The listing builds one solid part. Answer for the finished solid, in the listing's coordinates (mm). Give positions to 0.01 mm unless a question says otherwise; leave off trailing zeros. Order: outer loops, then holes, each group sorted by start corner. A loop starts at its lowest first (then second) coordinate and runs counter-clockwise, first axis right, second up. Notation, with made-up numbers: (28.5, -22) - (47.5, -22) arc R35 cw to (47.5, 12) - close; hole circle Ø10 at (31, 6). An arc over 180 degrees is marked (long way). Answer as a JSON object with one key per item and string values. Group by question number.
Q1. Consider line 1 (Z direction, x = 0, y = -1.25); line 2 (Z direction, x = -0.5, y = 0.75); line 3 (Y direction, x = -0.25, z = -29). Determine where each line is inside the solid, lowest interval first.
Q2. A cutting plane is placed at C-C, the plane z = -16. Give the vertices of the cut face in (x, y).
Q3. A cutting plane is placed at B-B, the plane y = -1.75. Give the vertices of the cut face in (x, z) (3 decimals), and give its area (3 significant figures).
Q4. Given pin 1 (2 mm diameter, centred on y = 1, z = 25.5, fed in from +X), flat-ended and moving along its own axis, determine where the tip first touches the part or whether it passes through.
Q5. A cutting plane is placed at A-A, the plane x = 0. Give the vertices of the cut face in (y, z), and give its area (3 significant figures).
Q6. The mould has two halves that part along X. Classify faces 1 (the face through (-3.946, 0.174, 0.64)), 2 (the face through (0.172, 0.055, 43.855)), 3 (the face through (0, 0, -45.72)): released by +X, released by -X, zero draft, split by the parting line, or undercut.
Autodesk Inventor part; units mm, degrees
ref_plane "YZ Plane" through (0, 0, 0) normal (1, 0, 0) x (0, 1, 0)
ref_plane "XZ Plane" through (0, 0, 0) normal (0, 1, 0) x (-1, 0, 0)
ref_plane "XY Plane" through (0, 0, 0) normal (0, 0, 1) x (1, 0, 0)
sketch "Sketch1" plane through (0, 0, 0) normal (0, 0, 1) x (1, 0, 0)
  circle A0 centre (0, 0) radius 3.9497
  dimension "d0" = 7.8994
extrude "Extrusion1" add sketch "Sketch1" against normal mid plane 91.44
sketch "Sketch2" plane through (0, 0, 0) normal (0, 1, 0) x (-1, 0, 0)
  circle A0 centre (0, 42.545) radius 1.3208
  line L0 (-3.9497, 45.72) -> (3.9497, 45.72)
  point P0 (0, 45.72)
  dimension "d3" = 2.6416
  dimension "d4" = 3.175
extrude "Extrusion2" cut sketch "Sketch2" along normal through all both and the other way through all
mirror "Mirror1" about plane through (0, 0, 0) normal (0, 0, 1) of "Extrusion2"
properties part number "Handle_Rod" material "Steel, Mild"
Reply:
{
 "1": {"line 1": "z = -45.72 to -43.87, -41.22 to 41.22, 43.87 to 45.72", "line 2": "z = -45.72 to -43.77, -41.32 to 41.32, 43.77 to 45.72", "line 3": "y = -3.94 to 3.94"},
 "2": {"outline": "circle Ø7.9 at (0, 0)"},
 "3": {"outline": "(-3.541, -45.72) - (3.541, -45.72) - (3.541, 45.72) - (-3.541, 45.72) - close; hole circle Ø2.642 at (0, -42.545); hole circle Ø2.642 at (0, 42.545)", "area": "637 mm^2"},
 "4": {"pin 1": "stops at x = 3.95"},
 "5": {"outline": "(-3.95, -45.72) - (3.95, -45.72) - (3.95, -43.87) - (-3.95, -43.87) - close; (-3.95, -41.22) - (3.95, -41.22) - (3.95, 41.22) - (-3.95, 41.22) - close; (-3.95, 43.87) - (3.95, 43.87) - (3.95, 45.72) - (-3.95, 45.72) - close", "area": "681 mm^2"},
 "6": {"face 1": "split by the parting line", "face 2": "undercut", "face 3": "zero draft"}
}
